from build123d import *

# Parameters (mm, degrees)
BOSS_EXTRUDE1_DEPTH = 25.4
SKETCH2_W           = 15.24
SKETCH2_H           = 10.16
CUT_EXTRUDE1_DEPTH  = 144.272


with BuildPart() as part:
    # Sketch1 → Boss-Extrude1 (new body)
    with BuildSketch(Plane(origin=(0, 0, 0), x_dir=(1, 0, 0), z_dir=(0, 1, 0))):
        with BuildLine():
            Line((-29.342474553, 61.985769231), (-28.255716236, 59.69))
            ThreePointArc((-28.255716236, 59.69), (0, 66.04), (28.255716236, 59.69))
            Line((28.255716236, 59.69), (29.342474553, 61.985769231))
            ThreePointArc((29.342474553, 61.985769231), (0, 68.58), (-29.342474553, 61.985769231))
        make_face()
    extrude(amount=BOSS_EXTRUDE1_DEPTH)

    # Sketch2 → Cut-Extrude1 (cut)
    with BuildSketch(Plane.XY):
        with Locations((0, 12.7)):
            Rectangle(SKETCH2_W, SKETCH2_H)
    extrude(amount=-CUT_EXTRUDE1_DEPTH, mode=Mode.SUBTRACT)


solid = part.part
Read the model definition and answer for the solid it produces. Units are mm, in the model's axes. A direction names the side the tool comes from. Round coordinates to 2 decimals unless told otherwise and drop trailing zeros. Loops run counter-clockwise (first coordinate to the right, second up) from the corner with the lowest first, then second, coordinate; pieces in that order, holes last.
Q1. Determine the mould class of faces 3 (the face through (0, 0, -67)), 4 (the face through (-28.807, 12.522, -60.854)), 5 (the face through (0, 25.4, -67)), 6 (the face through (-7.62, 13, -67)) for opening direction Y: released by +Y, released by -Y, zero draft, split by the parting line, or undercut.
Q2. Which of the six approach directions +Z, -Z, +X, -X, +Y, -Y give full straight-line access (tool end or side, diameter ignored) to faces 1 (the face through (0, 17.78, -67)), 2 (the face through (-0.41, 18.17, -66.04))?
Q3. Section C-C on z = -67.25 is taken. Write down the section's boundary in (x, y).
Q4. Each of these flat-tipped pins is pushed along its axis until it touches: pin 1 (4 mm diameter, centred on x = -15, y = 20.5, fed in from +Z); pin 2 (3 mm diameter, centred on y = 9.5, z = -61, fed in from +X); pin 3 (2 mm diameter, centred on y = 10, z = -64, fed in from -X). Where does it stop, or does it pass through?
Q5. Section A-A on y = 8.5 is taken. Write down the section's boundary in (x, z).
Q6. Section B-B on z = -60.25 is taken. Write down the section's boundary in (x, y).
Q7. Consider probe 1 along X at (y, z) = (8.75, -60.25); probe 2 along X at (y, z) = (12.25, -61.25); probe 3 along Z at (x, y) = (1, 23.75). Determine where each line is inside the solid, lowest interval first.
Q8. Section D-D on x = 14 is taken. Write down the section's boundary in (y, z), and give its area (3 significant figures).
Output:
1. face 3: released by -Y
1. face 4: zero draft
1. face 5: released by +Y
1. face 6: undercut
2. face 1: +Z, -Z
2. face 2: +Z, +Y, -Y
3. outline: (-13.44, 0) - (13.44, 0) - (13.44, 25.4) - (-13.44, 25.4) - close; hole (-7.62, 7.62) - (7.62, 7.62) - (7.62, 17.78) - (-7.62, 17.78) - close
4. pin 1: stops at z = -63.81
4. pin 2: stops at x = 29.34
4. pin 3: stops at x = -27.1
5. outline: (-29.34, -61.99) arc R68.58 ccw to (-7.62, -68.16) - (-7.62, -65.6) arc R66.04 cw to (-28.26, -59.69) - close; (7.62, -68.16) arc R68.58 ccw to (29.34, -61.99) - (28.26, -59.69) arc R66.04 cw to (7.62, -65.6) - close
6. outline: (-28.52, 0) - (-27.04, 0) - (-27.04, 25.4) - (-28.52, 25.4) - close; (27.04, 0) - (28.52, 0) - (28.52, 25.4) - (27.04, 25.4) - close
7. probe 1: x = -28.52 to -27.04, 27.04 to 28.52
7. probe 2: x = -28.99 to -24.69, 24.69 to 28.99
7. probe 3: z = -68.57 to -66.03
8. outline: (0, -67.14) - (25.4, -67.14) - (25.4, -64.54) - (0, -64.54) - close
8. area: 66.0 mm2
